```python
from build123d import *

# Parameters (mm, degrees)
SKETCH1_W                      = 150
SKETCH1_H                      = 200
BASE_FLANGE1_DEPTH             = 2
EDGE_FLANGE1_STRIP_W           = 28
EDGE_FLANGE1_STRIP_H           = 2
EDGE_FLANGE1_STRIP_CUT_DEPTH   = 200
EDGE_FLANGE1_STRIP_2_W         = 28
EDGE_FLANGE1_STRIP_2_H         = 2
EDGE_FLANGE1_STRIP_CUT_2_DEPTH = 200
EDGE_FLANGE1_DEPTH             = 200
EDGE_FLANGE1_BEND_DEPTH        = 200
SKETCH15_OUTSIDE_W             = 260.93
SKETCH15_OUTSIDE_H             = 212.93
SKETCH15_OUTSIDE_R             = 8
CUT_EXTRUDE1_DEPTH             = 238.099135384
SKETCH16_R                     = 5
CUT_EXTRUDE2_DEPTH             = 197.033160551


# Sheet-metal steps are written as plain solids
with BuildPart() as part:
    # Sketch1 → Base-Flange1 (new body)
    with BuildSketch(Plane(origin=(0, 0, 0), x_dir=(1, 0, 0), z_dir=(0, 1, 0))):
        Rectangle(SKETCH1_W, SKETCH1_H)
    extrude(amount=-BASE_FLANGE1_DEPTH)

    # Edge-Flange1 strip (across the edge) → Edge-Flange1 strip cut (cut)
    with BuildSketch(Plane(origin=(75, 0, 100), x_dir=(-1, 0, 0), z_dir=(0, 0, -1))):
        with Locations((-4, -1)):
            Rectangle(EDGE_FLANGE1_STRIP_W, EDGE_FLANGE1_STRIP_H)
    extrude(amount=EDGE_FLANGE1_STRIP_CUT_DEPTH, mode=Mode.SUBTRACT)

    # Edge-Flange1 strip 2 (across the edge) → Edge-Flange1 strip cut 2 (cut)
    with BuildSketch(Plane(origin=(-75, 0, -100), x_dir=(1, 0, 0), z_dir=(0, 0, 1))):
        with Locations((-4, -1)):
            Rectangle(EDGE_FLANGE1_STRIP_2_W, EDGE_FLANGE1_STRIP_2_H)
    extrude(amount=EDGE_FLANGE1_STRIP_CUT_2_DEPTH, mode=Mode.SUBTRACT)

    # Edge-Flange1 section (across the edge) → Edge-Flange1 (add)
    with BuildSketch(Plane(origin=(75, 0, 100), x_dir=(-1, 0, 0), z_dir=(0, 0, -1))):
        with BuildLine():
            Line((-2, 10), (-2, 150))
            Line((-2, 150), (0, 150))
            Line((0, 150), (0, 10))
            ThreePointArc((0, 10), (2.928932188, 2.928932188), (10, 0))
            Line((10, 0), (10, -2))
            ThreePointArc((10, -2), (1.514718626, 1.514718626), (-2, 10))
        make_face()
    extrude(amount=EDGE_FLANGE1_DEPTH)

    # Edge-Flange1 section 2 (across the edge) → Edge-Flange1 bend (add)
    with BuildSketch(Plane(origin=(-75, 0, -100), x_dir=(1, 0, 0), z_dir=(0, 0, 1))):
        with BuildLine():
            Line((-2, 10), (-2, 150))
            Line((-2, 150), (0, 150))
            Line((0, 150), (0, 10))
            ThreePointArc((0, 10), (2.928932188, 2.928932188), (10, 0))
            Line((10, 0), (10, -2))
            ThreePointArc((10, -2), (1.514718626, 1.514718626), (-2, 10))
        make_face()
    extrude(amount=EDGE_FLANGE1_BEND_DEPTH)

    # Sketch15 outside → Cut-Extrude1 (cut, through all)
    # profile 1 of 4: a face of its own
    with BuildSketch(Plane.ZY.offset(77)):
        with Locations((0, 74)):
            Rectangle(SKETCH15_OUTSIDE_W, SKETCH15_OUTSIDE_H)
        with BuildLine():
            Line((-1.916529607, 141.180744276), (73.507242037, 89.243178795))
            ThreePointArc((73.507242037, 89.243178795), (78.277963521, 83.867184852), (80, 76.888955512))
            Line((80, 76.888955512), (80, 20))
            ThreePointArc((80, 20), (82.928932188, 12.928932188), (90, 10))
            Line((90, 10), (95, 10))
            ThreePointArc((95, 10), (98.535533906, 8.535533906), (100, 5))
            Line((100, 5), (100, -2))
            Line((100, -2), (-100, -2))
            Line((-100, -2), (-100, 99))
            Line((-100, 99), (-100, 120))
            ThreePointArc((-100, 120), (-91.213203436, 141.213203436), (-70, 150))
            Line((-70, 150), (-49, 150))
            Line((-49, 150), (-30.274003064, 150))
            ThreePointArc((-30.274003064, 150), (-15.425387199, 147.744304445), (-1.916529607, 141.180744276))
        make_face(mode=Mode.SUBTRACT)
    # profile 2 of 4: a face of its own
    with BuildSketch(Plane.ZY.offset(77)):
        with Locations(Location((61, 35, 0), (0, 0, 270))):
            Circle(SKETCH15_OUTSIDE_R)
    # profile 3 of 4: a face of its own
    with BuildSketch(Plane.ZY.offset(77)):
        with Locations(Location((-70, 120, 0), (0, 0, 270))):
            Circle(SKETCH15_OUTSIDE_R)
    # profile 4 of 4: a face of its own
    with BuildSketch(Plane.ZY.offset(77)):
        with Locations(Location((5, 35, 0), (0, 0, 270))):
            Circle(SKETCH15_OUTSIDE_R)
    extrude(amount=-CUT_EXTRUDE1_DEPTH, mode=Mode.SUBTRACT)

    # Sketch16 → Cut-Extrude2 (cut, through all)
    with BuildSketch(Plane(origin=(0, 0, 0), x_dir=(1, 0, 0), z_dir=(0, 1, 0))):
        with Locations(Location((-47, 75, 0), (0, 0, 270))):
            Circle(SKETCH16_R)
        with Locations(Location((47, 75, 0), (0, 0, 90))):
            Circle(SKETCH16_R)
        with Locations(Location((47, -75, 0), (0, 0, 270))):
            Circle(SKETCH16_R)
        with Locations(Location((-47, -75, 0), (0, 0, 90))):
            Circle(SKETCH16_R)
        with BuildLine():
            Line((7.5, 20), (7.5, -20))
            ThreePointArc((7.5, -20), (0, -27.5), (-7.5, -20))
            Line((-7.5, -20), (-7.5, 20))
            ThreePointArc((-7.5, 20), (0, 27.5), (7.5, 20))
        make_face()
    extrude(amount=-CUT_EXTRUDE2_DEPTH, mode=Mode.SUBTRACT)


solid = part.part
```
The listing builds one solid part. Answer for the finished solid, in the listing's coordinates (mm). A direction names the side the tool comes from. Give positions to 0.01 mm unless a question says otherwise; leave off trailing zeros. Order: outer loops, then holes, each group sorted by start corner. A loop starts at its lowest first (then second) coordinate and runs counter-clockwise, first axis right, second up. Notation, with made-up numbers: (45, 25.25) - (58, 25.25) arc R13 ccw to (58, 29.25) - close; hole circle Ø1 at (32.25, 50.5). An arc over 180 degrees is marked (long way). Use one line per item in the form item = value. Start each with the question number.
(1) A cutting plane is placed at B-B, the plane x = 0. Write down the section's boundary in (y, z).
(2) Flat-ended cylindrical pins translate along their axes: pin 1 Ø1.6 at (x, y) = (76, 59) entering from +Z; pin 2 Ø5 at (x, z) = (-12.5, -47) entering from +Y; pin 3 Ø18.5 at (y, z) = (35, 5) entering from -X; pin 4 Ø1 at (x, z) = (-76.5, 92.5) entering from +Y. Find the tip coordinate at first contact, or state that the pin passes through.
(3) Consider line 1 (Z direction, x = -76.4, y = 35); line 2 (X direction, y = 96, z = -66); line 3 (Y direction, x = 26, z = 90). Determine where each line is inside the solid, lowest interval first. Write a range as from..to.
(4) For faces 1 (the cylindrical face through (75.986, 36.041, 68.932)), 2 (the cylindrical face through (0.16, -0.99, 27.5)), determine the directions among +Z, -Z, +X, -X, +Y, -Y from which every point of the face is accessible in a straight line to the end or side of a thin tool.
(5) The mould has two halves that part along Z. Classify faces 3 (the flat face through (-15, 0, -1)), 4 (the cylindrical face through (43, -1, -78)), 5 (the cylindrical face through (75.986, 140.979, -91.445)): released by +Z, released by -Z, zero draft, split by the parting line, or undercut.
(6) A cutting plane is placed at A-A, the plane y = 35. Write down the section's boundary in (x, z).
(7) A cutting plane is placed at C-C, the plane z = -75. Write down the section's boundary in (x, y) (3 decimals), then the cut area to 3 significant figures.
(8) A cutting plane is placed at D-D, the plane x = -47. Write down the section's boundary in (y, z).
Ans:
q1.outline = (-2, -100) - (0, -100) - (0, -27.5) - (-2, -27.5) - close; (-2, 27.5) - (0, 27.5) - (0, 100) - (-2, 100) - close
q2.pin_1 = 80
q2.pin_2 = 0
q2.pin_3 = -77
q2.pin_4 = 10
q3.line_1 = -100..-3, 13..53, 69..80
q3.line_2 = -77..-75, 75..77
q3.line_3 = -2..0
q4.face_1 = +X, -X
q4.face_2 = +Y, -Y
q5.face_3 = zero draft
q5.face_4 = undercut
q5.face_5 = released by -Z
q6.outline = (-77, -100) - (-75, -100) - (-75, -3) - (-77, -3) - close; (-77, 13) - (-75, 13) - (-75, 53) - (-77, 53) - close; (-77, 69) - (-75, 69) - (-75, 80) - (-77, 80) - close; (75, -100) - (77, -100) - (77, -3) - (75, -3) - close; (75, 13) - (77, 13) - (77, 53) - (75, 53) - close; (75, 69) - (77, 69) - (77, 80) - (75, 80) - close
q7.outline = (-77, 10) arc R12 ccw to (-65, -2) - (-52, -2) - (-52, 0) - (-65, 0) arc R10 cw to (-75, 10) - (-75, 113.755) - (-77, 113.755) - close; (-77, 126.245) - (-75, 126.245) - (-75, 149.58) - (-77, 149.58) - close; (-42, -2) - (42, -2) - (42, 0) - (-42, 0) - close; (52, -2) - (65, -2) arc R12 ccw to (77, 10) - (77, 113.755) - (75, 113.755) - (75, 10) arc R10 cw to (65, 0) - (52, 0) - close; (75, 126.245) - (77, 126.245) - (77, 149.58) - (75, 149.58) - close
q7.area = 797 mm^2
q8.outline = (-2, -100) - (0, -100) - (0, -80) - (-2, -80) - close; (-2, -70) - (0, -70) - (0, 70) - (-2, 70) - close; (-2, 80) - (0, 80) - (0, 100) - (-2, 100) - close
